Job drawing, mm, ordinate dimensions from the low corner. One solid piece. A direction names the side the tool comes from. Give positions to 0.01 mm unless a question says otherwise; leave off trailing zeros. Loops run counter-clockwise (first coordinate to the right, second up) from the corner with the lowest first, then second, coordinate; pieces in that order, holes last. Notation, with made-up numbers: M 6,-30 L 26,-30 A20 ccw 26,4 Z; hole C -34,87.5 d4. An arc over 180 degrees is marked long. One line per question, with ' | ' between items.
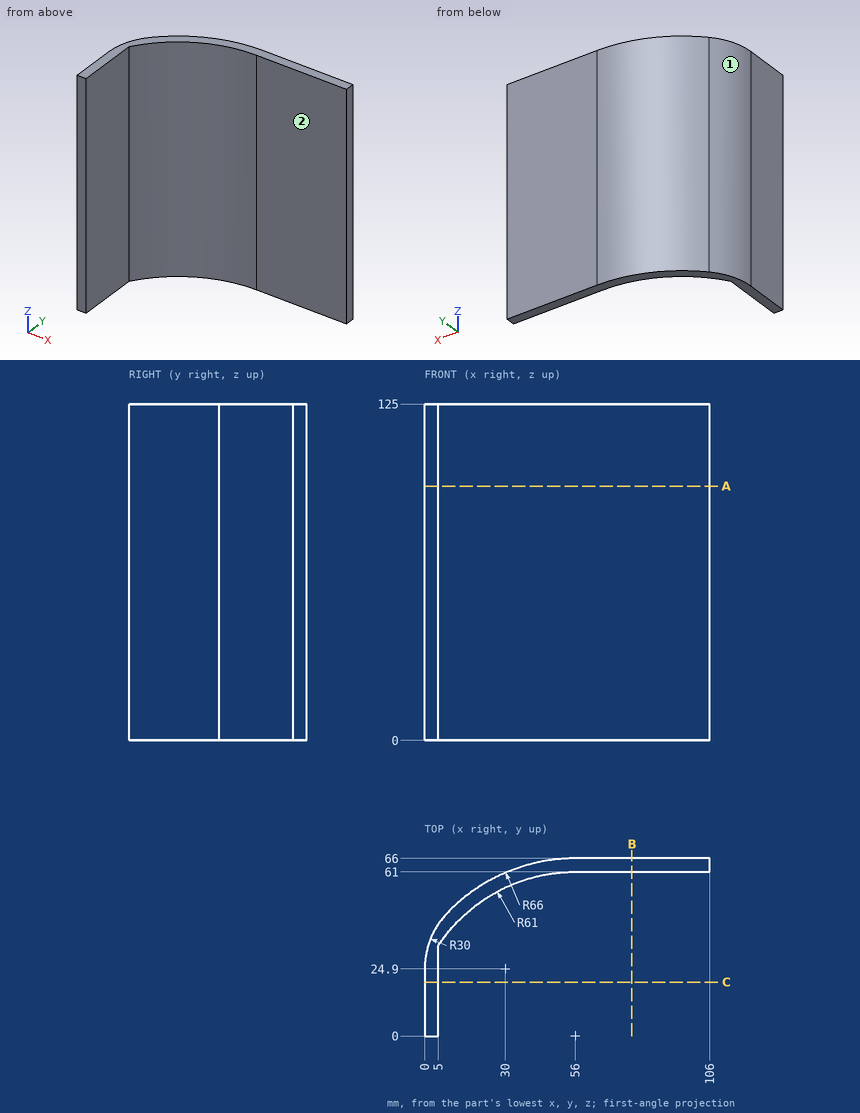
Item 1: Drill centre lines: line 1 along X through (y, z) = (19, 88); line 2 along Y through (x, z) = (89.5, 21); line 3 along Y through (x, z) = (16, 61.5) (1 decimal). Where is each one in solid material? Low to high. Write a range as [from, to].
Conclusion:
line 1: [0, 5] | line 2: [61, 66] | line 3: [46.1, 52.5]
Item 2: Saw through at C-C on y = 20. Give the cut face in (x, z), and give its area (3 significant figures).
Conclusion:
outline: M 0,0 L 5,0 L 5,125 L 0,125 Z | area: 625 mm²
Item 3: Saw through at A-A on z = 94.5. Give the cut face in (x, y), and give its area (3 significant figures).
Conclusion:
outline: M 0,0 L 5,0 L 5,33.47 A61 cw 56,61 L 106,61 L 106,66 L 56,66 A66 ccw 8.33,45.65 A30 ccw 0,24.9 Z | area: 727 mm²
Item 4: Saw through at B-B on x = 77. Give the cut face in (y, z), and give its area (3 significant figures).
Conclusion:
outline: M 61,0 L 66,0 L 66,125 L 61,125 Z | area: 625 mm²
Item 5: Drop flat-ended pins along their axis: P1, Ø1.5, axis at y = 19.5, z = 27.5, coming from the +X side; P2, Ø4, axis at x = 55.5, z = 77, coming from the -Y side; P3, Ø2, axis at y = 14.5, z = 105.5, coming from the -X side; P4, Ø10, axis at x = 36.5, z = 15, coming from the +Y side. Give the stop position or say it passes through.
Conclusion:
P1: x = 5 | P2: y = 60.95 | P3: x = 0 | P4: y = 64.39
Item 6: 3-axis set-ups, long thin cutter, end or side, ignore diameter. For the marked faces 1 and 2: which of +Z, -Z, +X, -X, +Y, -Y reach the whole face in a straight line?
Conclusion:
face 1: +Z, -Z, -X, +Y | face 2: +Z, -Z, +X, -Y
